Could you check a few things on this drawing? It's one solid part, dimensions in mm from its lowest x, y, z. Round coordinates to 2 decimals unless told otherwise and drop trailing zeros. Loops run counter-clockwise (first coordinate to the right, second up) from the corner with the lowest first, then second, coordinate; pieces in that order, holes last. Notation, with made-up numbers: M 84.5,-23.5 L 121.5,-23.5 A7 cw 121.5,-18.5 Z; hole C 64.25,0.5 d11. An arc over 180 degrees is marked long. Write each question's results on one line, items separated by ' | '. Start each with the question number.
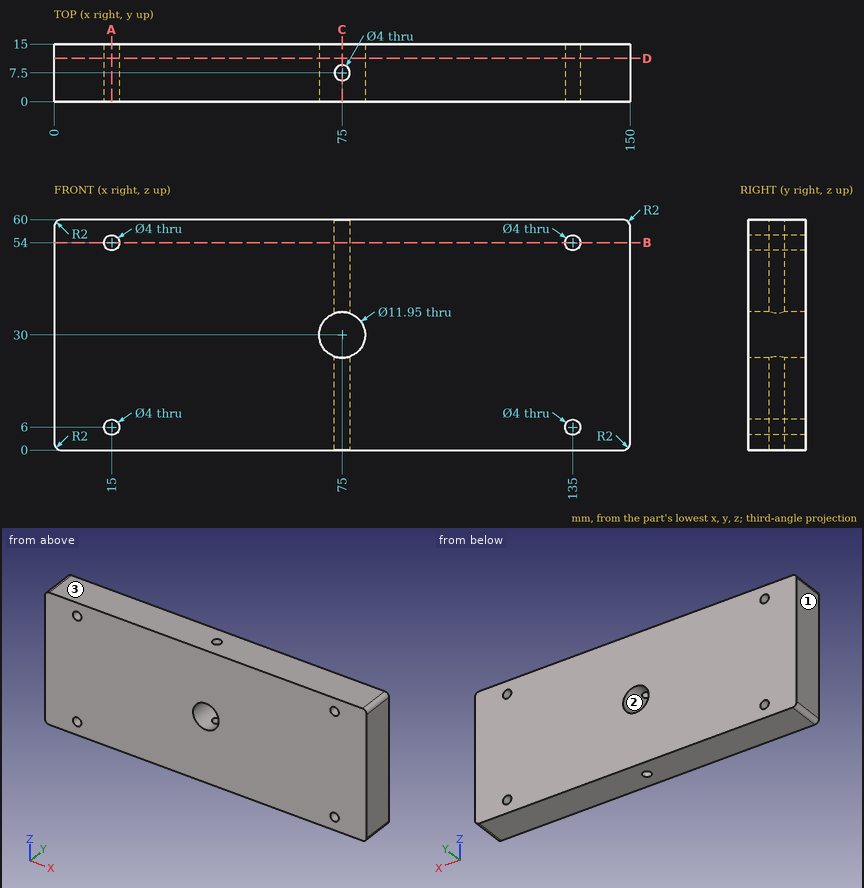
1. If we mould it in two halves opening along Z, with no side actions, what happens to the marked faces 1, 2 and 3? For each: released by +Z, released by -Z, zero draft, split by the parting line, or undercut.
2. I want a section at B-B on z = 54. List the corners of the cut face in (x, y) for me.
3. I need wall thicknesses on line 1 along X through (y, z) = (11.5, 6); line 2 along Z through (x, y) = (16, 13.5); line 3 along Z through (x, y) = (135.5, 13.5). Which ranges of each line are inside material? Lowest first, please.
4. I want a section at D-D on y = 11.25. List the corners of the cut face in (x, z) for me (3 decimals), plus the area to 3 significant figures.
5. For pin 1 (5 mm diameter, centred on x = 75, y = 7.5, fed in from -Z), with a flat end and sliding along its axis, tell me the tip position at first contact or that it passes through.
6. I want a section at C-C on x = 75. List the corners of the cut face in (y, z) for me (3 decimals), plus the area to 3 significant figures.
7. I want a section at A-A on x = 15. List the corners of the cut face in (y, z) for me.
Outcome:
1) face 1: zero draft | face 2: undercut | face 3: released by +Z
2) outline: M 0,0 L 13,0 L 13,15 L 0,15 Z; M 17,0 L 133,0 L 133,15 L 17,15 Z; M 137,0 L 150,0 L 150,15 L 137,15 Z; hole C 75,7.5 d4
3) line 1: 0 to 13, 17 to 133, 137 to 150 | line 2: 0 to 4.27, 7.73 to 52.27, 55.73 to 60 | line 3: 0 to 4.06, 7.94 to 52.06, 55.94 to 60
4) outline: M 0,2 A2 ccw 2,0 L 148,0 A2 ccw 150,2 L 150,58 A2 ccw 148,60 L 2,60 A2 ccw 0,58 Z; hole C 15,6 d4; hole C 15,54 d4; hole C 75,30 d11.95; hole C 135,6 d4; hole C 135,54 d4 | area: 8,830 mm2
5) pin 1: z = 0
6) outline: M 0,0 L 5.5,0 L 5.5,24.025 L 0,24.025 Z; M 0,35.975 L 5.5,35.975 L 5.5,60 L 0,60 Z; M 9.5,0 L 15,0 L 15,24.025 L 9.5,24.025 Z; M 9.5,35.975 L 15,35.975 L 15,60 L 9.5,60 Z | area: 529 mm2
7) outline: M 0,0 L 15,0 L 15,4 L 0,4 Z; M 0,8 L 15,8 L 15,52 L 0,52 Z; M 0,56 L 15,56 L 15,60 L 0,60 Z
